```python
from build123d import *

# Parameters (mm, degrees)
F0_W     = 35
F0_H     = 25
F0_R     = 1.6
F0_W_2   = 19.1
F0_H_2   = 19.1
F1_DEPTH = 4.1
F2_W     = 35
F2_H     = 25
F2_R     = 3.1
F2_W_2   = 17.4
F2_H_2   = 17.4
F3_DEPTH = 14.1


with BuildPart() as f1:
    # F0 (on Front) → F1 (new body)
    with BuildSketch(Plane.XZ):
        Rectangle(F0_W, F0_H)
        with Locations((-13, 0)):
            Circle(F0_R, mode=Mode.SUBTRACT)
        Rectangle(F0_W_2, F0_H_2, mode=Mode.SUBTRACT)
        with Locations((13, 0)):
            Circle(F0_R, mode=Mode.SUBTRACT)
    extrude(amount=F1_DEPTH)

    # F2 (on face) → F3 (join)
    with BuildSketch(Plane.XZ.offset(4.1)):
        Rectangle(F2_W, F2_H)
        with Locations((-13, 0)):
            Circle(F2_R, mode=Mode.SUBTRACT)
        Rectangle(F2_W_2, F2_H_2, mode=Mode.SUBTRACT)
        with Locations((13, 0)):
            Circle(F2_R, mode=Mode.SUBTRACT)
    extrude(amount=F3_DEPTH)


solid = f1.part
```
The listing builds one solid part. Answer for the finished solid, in the listing's coordinates (mm). A direction names the side the tool comes from. Give positions to 0.01 mm unless a question says otherwise; leave off trailing zeros. Loops run counter-clockwise (first coordinate to the right, second up) from the corner with the lowest first, then second, coordinate; pieces in that order, holes last. Notation, with made-up numbers: (45, 42.25) - (69, 42.25) arc R16 cw to (69, 66.25) - close; hole circle Ø6 at (25, 66.25). An arc over 180 degrees is marked (long way). Answer as CSV lines item,"result". Start each with the question number.
Item 1: The mould has two halves that part along Z. Classify faces 4 (the face through (-8.7, -11, 0)), 5 (the face through (0, -9, -12.5)), 6 (the face through (0, -18.2, 11)): +Z half, -Z half, draft (parallel to the pull), parting line (faces both ways), or undercut.
Item 2: A cutting plane is placed at D-D on z = 3.75. Determine the outline of the cut face in (x, y), then the cut area to 3 significant figures.
Item 3: For faces 1 (the face through (0, -2, -9.55)), 2 (the face through (0, -11, -8.7)), 3 (the face through (-11.7, -4.1, -1.3)), determine the directions among +Z, -Z, +X, -X, +Y, -Y from which every point of the face is accessible in a straight line to the end or side of a thin tool.
Item 4: Find the intervals of material crossed by line 1 (X direction, y = -4.5, z = 5); line 2 (Z direction, x = -8, y = -8.25); line 3 (X direction, y = -1, z = -5.5), in increasing order. Write a range as from..to.
Item 5: Each of these flat-tipped pins is pushed along its axis until it touches: pin 1 (7 mm diameter, centred on x = 12, z = -0.5, fed in from -Y); pin 2 (5 mm diameter, centred on x = -13, z = 0, fed in from -Y). Where does it stop, or does it pass through?
Item 6: A cutting plane is placed at A-A on x = -13. Determine the outline of the cut face in (y, z), then the cut area to 3 significant figures.
Item 7: A cutting plane is placed at C-C on y = -1.25. Determine the outline of the cut face in (x, z).
Item 8: A cutting plane is placed at B-B on z = 0. Determine the outline of the cut face in (x, y).
Found:
1,face 4,"undercut"
1,face 5,"-Z half"
1,face 6,"draft"
2,outline,"(-17.5, -18.2) - (-8.7, -18.2) - (-8.7, -4.1) - (-9.55, -4.1) - (-9.55, 0) - (-17.5, 0) - close; (8.7, -18.2) - (17.5, -18.2) - (17.5, 0) - (9.55, 0) - (9.55, -4.1) - (8.7, -4.1) - close"
2,area,"313 mm^2"
3,face 1,"+Y"
3,face 2,"+Y, -Y"
3,face 3,"-Y"
4,line 1,"x = -17.5..-8.7, 8.7..17.5"
4,line 2,"z = -12.5..-8.7, 8.7..12.5"
4,line 3,"x = -17.5..-9.55, 9.55..17.5"
5,pin 1,"stops at y = -18.2"
5,pin 2,"stops at y = -4.1"
6,outline,"(-18.2, -12.5) - (0, -12.5) - (0, -1.6) - (-4.1, -1.6) - (-4.1, -3.1) - (-18.2, -3.1) - close; (-18.2, 3.1) - (-4.1, 3.1) - (-4.1, 1.6) - (0, 1.6) - (0, 12.5) - (-18.2, 12.5) - close"
6,area,"354 mm^2"
7,outline,"(-17.5, -12.5) - (17.5, -12.5) - (17.5, 12.5) - (-17.5, 12.5) - close; hole circle Ø3.2 at (-13, 0); hole (-9.55, -9.55) - (9.55, -9.55) - (9.55, 9.55) - (-9.55, 9.55) - close; hole circle Ø3.2 at (13, 0)"
8,outline,"(-17.5, -18.2) - (-16.1, -18.2) - (-16.1, -4.1) - (-14.6, -4.1) - (-14.6, 0) - (-17.5, 0) - close; (-11.4, -4.1) - (-9.9, -4.1) - (-9.9, -18.2) - (-8.7, -18.2) - (-8.7, -4.1) - (-9.55, -4.1) - (-9.55, 0) - (-11.4, 0) - close; (8.7, -18.2) - (9.9, -18.2) - (9.9, -4.1) - (11.4, -4.1) - (11.4, 0) - (9.55, 0) - (9.55, -4.1) - (8.7, -4.1) - close; (14.6, -4.1) - (16.1, -4.1) - (16.1, -18.2) - (17.5, -18.2) - (17.5, 0) - (14.6, 0) - close"
